Part model, mm, in its own coordinate system. A direction names the side the tool comes from. Coordinates: 2 decimals unless noted, no trailing zeros. Loops run counter-clockwise (first coordinate to the right, second up) from the corner with the lowest first, then second, coordinate; pieces in that order, holes last. Notation, with made-up numbers: (21.25, -0.75) - (80.25, -0.75) arc R20 cw to (80.25, 4.25) - close; hole circle Ø2 at (43, 80). An arc over 180 degrees is marked (long way). Use a Markdown table: item, result. Add a question column.
1. Wall check: probe 1 along Z at (x, y) = (23, 1); probe 2 along X at (y, z) = (-1.75, 1); probe 3 along Z at (x, y) = (0, 1). Give the ranges that are in metal, low to high. Write a range as [from, to].
2. Band-saw the part on B-B, the plane x = 0. Give the cut face in (y, z).
3. Band-saw the part on A-A, the plane z = 3.5. Give the cut face in (x, y).
4. Drop flat-ended pins along their axis: pin 1 (11.5 mm diameter, centred on x = 0, z = 3.5, fed in from +Y); pin 2 (6 mm diameter, centred on y = 5, z = 13, fed in from -X); pin 3 (4.5 mm diameter, centred on x = -23, z = -14.5, fed in from +Y); pin 4 (3.5 mm diameter, centred on x = 23, y = -1.5, fed in from +Z). Give the stop position or say it passes through.
5. Pull direction X, two halves, no side cores. Call faces 4 (the flat face through (17, 0, 14)), 5 (the flat face through (23, 0, 11)), 6 (the cylindrical face through (20.253, -0.14, 3.621)), 7 (the cylindrical face through (-25.747, -0.14, -14.379)): pulls with the +X half, pulls with the -X half, needs draft (parallel to the pull), parting line crosses it, or undercut.
6. 3-axis set-ups, long thin cutter, end or side, ignore diameter. For faces 1 (the flat face through (5, -1, 1)), 2 (the flat face through (-17, 0, 14)), 3 (the cylindrical face through (-25.747, -0.14, 3.621)): which of +Z, -Z, +X, -X, +Y, -Y reach the whole face in a straight line?
7. Band-saw the part on C-C, the plane z = -14.5. Give the cut face in (x, y).
8. Band-saw the part on D-D, the plane x = -23. Give the cut face in (y, z).
from build123d import *

# Parameters (mm, degrees)
F1_DEPTH = 10
F2_R     = 5
F2_R_2   = 2.75
F3_DEPTH = 20
F4_SIZE  = 5
F5_SIZE  = 2
F6_R     = 10
F7_DEPTH = 11


with BuildPart() as f1:
    # F0 (on Front) → F1 (new body, symmetric)
    with BuildSketch(Plane.XZ):
        Polygon((17, 11), (17, 21.5), (-17, 21.5), (-17, 11), (-30, 11), (-30, -21.5), (30, -21.5), (30, 11), align=None)
    extrude(amount=F1_DEPTH, both=True)

    # F2 (on face) → F3 (cut)
    with BuildSketch(Plane.XZ.offset(10)):
        with Locations((0, 3.5)):
            Circle(F2_R)
        with Locations((23, 3.5)):
            Circle(F2_R_2)
        with Locations((23, -14.5)):
            Circle(F2_R_2)
        with Locations((-23, -14.5)):
            Circle(F2_R_2)
        with Locations((-23, 3.5)):
            Circle(F2_R_2)
    extrude(amount=-F3_DEPTH, mode=Mode.SUBTRACT)

    # F4
    f4_edges = [f1.edges().sort_by_distance(p)[0] for p in [
        (-17, 0, 21.5),
        (17, 0, 21.5),
    ]]
    chamfer(f4_edges, length=F4_SIZE)

    # F5
    f5_edges = [f1.edges().sort_by_distance(p)[0] for p in [
        (30, 0, 11),
        (-30, 0, 11),
    ]]
    chamfer(f5_edges, length=F5_SIZE)

    # F6 (on face) → F7 (cut)
    with BuildSketch(Plane(origin=(0, 10, 0), x_dir=(-1, 0, 0), z_dir=(0, 1, 0))):
        with Locations((0, 3.5)):
            Circle(F6_R)
    extrude(amount=-F7_DEPTH, mode=Mode.SUBTRACT)


solid = f1.part
Geometry check:
| question | item | result |
|---|---|---|
| 1 | probe 1 | z = [-21.5, -17.25], [-11.75, 0.75], [6.25, 11] |
| 1 | probe 2 | x = [-30, -24.15], [-21.85, -4.33], [4.33, 21.85], [24.15, 30] |
| 1 | probe 3 | z = [-21.5, -6.5], [13.5, 21.5] |
| 2 | outline | (-10, -21.5) - (10, -21.5) - (10, -6.5) - (-1, -6.5) - (-1, -1.5) - (-10, -1.5) - close; (-10, 8.5) - (-1, 8.5) - (-1, 13.5) - (10, 13.5) - (10, 21.5) - (-10, 21.5) - close |
| 3 | outline | (-30, -10) - (-25.75, -10) - (-25.75, 10) - (-30, 10) - close; (-20.25, -10) - (-5, -10) - (-5, -1) - (-10, -1) - (-10, 10) - (-20.25, 10) - close; (5, -10) - (20.25, -10) - (20.25, 10) - (10, 10) - (10, -1) - (5, -1) - close; (25.75, -10) - (30, -10) - (30, 10) - (25.75, 10) - close |
| 4 | pin 1 | stops at y = -1 |
| 4 | pin 2 | stops at x = -29 |
| 4 | pin 3 | passes through |
| 4 | pin 4 | stops at z = 11 |
| 5 | face 4 | pulls with the +X half |
| 5 | face 5 | needs draft |
| 5 | face 6 | undercut |
| 5 | face 7 | undercut |
| 6 | face 1 | +Y |
| 6 | face 2 | +Z, -X, +Y, -Y |
| 6 | face 3 | +Y, -Y |
| 7 | outline | (-30, -10) - (-25.75, -10) - (-25.75, 10) - (-30, 10) - close; (-20.25, -10) - (20.25, -10) - (20.25, 10) - (-20.25, 10) - close; (25.75, -10) - (30, -10) - (30, 10) - (25.75, 10) - close |
| 8 | outline | (-10, -21.5) - (10, -21.5) - (10, -17.25) - (-10, -17.25) - close; (-10, -11.75) - (10, -11.75) - (10, 0.75) - (-10, 0.75) - close; (-10, 6.25) - (10, 6.25) - (10, 11) - (-10, 11) - close |
